Here's how the part is built. I have some questions about the finished solid (model axes, mm). Coordinates: 2 decimals unless noted, no trailing zeros. Order: outer loops, then holes, each group sorted by start corner. A loop starts at its lowest first (then second) coordinate and runs counter-clockwise, first axis right, second up. Notation, with made-up numbers: (24.25, -1) - (83.25, -1) arc R22 ccw to (83.25, 18) - close; hole circle Ø5 at (42, 13.25). An arc over 180 degrees is marked (long way). Answer in a Markdown table with one row per item. Add a question column.
Item 1: I want a section at B-B (y = 1.8). Please give me the cut outline in (x, z) (3 decimals).
Item 2: I want a section at D-D (x = 49). Please give me the cut outline in (y, z) (3 decimals).
Item 3: I want a section at C-C (z = -168). Please give me the cut outline in (x, y) (3 decimals).
Item 4: Will these pins go through, and if not, where does the flat tip stop? pin 1 Ø1 at (y, z) = (1, -153.5) entering from +X; pin 2 Ø1 at (y, z) = (1, -146.5) entering from +X; pin 3 Ø8 at (x, z) = (265.28, -74.56) entering from -Y.
Item 5: I want a section at A-A (x = 224.75). Please give me the cut outline in (y, z) (3 decimals).
Item 6: If I drill on line 1 along Z through (x, y) = (389, 1.45); line 2 along X through (y, z) = (0.75, -97); line 3 along X through (y, z) = (0.65, -95.5), over which ranges is the centre line in solid material (lowest first)? Write a range as from..to.
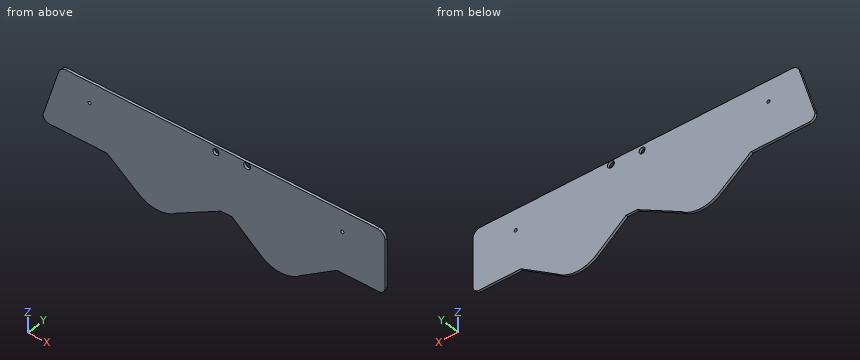
```python
from build123d import *

# Parameters (mm, degrees)
SKETCH1_R           = 3.716178426
SKETCH1_R_2         = 4.313560469
SKETCH1_R_3         = 4.511205791
BOSS_EXTRUDE1_DEPTH = 3.175
SKETCH2_W           = 597.466303312
SKETCH2_H           = 60.972543052
CUT_EXTRUDE1_DEPTH  = 70
FILLET1_R           = 10
FILLET2_R           = 10
SKETCH3_R           = 3.990837639
CUT_EXTRUDE2_DEPTH  = 10
SKETCH4_R           = 2
CUT_EXTRUDE3_DEPTH  = 470.13785887
SKETCH5_R           = 2
CUT_EXTRUDE4_DEPTH  = 10
SKETCH6_R           = 40
BOSS_EXTRUDE2_DEPTH = 3.175
BOSS_EXTRUDE3_DEPTH = 3.175
SKETCH9_R           = 40
BOSS_EXTRUDE4_DEPTH = 3.175
BOSS_EXTRUDE6_DEPTH = 3.175


with BuildPart() as part:
    # Sketch1 → Boss-Extrude1 (new body)
    with BuildSketch(Plane(origin=(0, 0, 0), x_dir=(1, 0, 0), z_dir=(0, 1, 0))):
        with BuildLine():
            ThreePointArc((8, 150), (2.343145751, 147.656854249), (0, 142))
            Line((0, 142), (42, 8))
            ThreePointArc((42, 8), (44.343145751, 2.343145751), (50, 0))
            Line((50, 0), (436.5, 0))
            ThreePointArc((436.5, 0), (442.156854249, 2.343145751), (444.5, 8))
            Line((444.5, 8), (444.5, 142))
            ThreePointArc((444.5, 142), (442.156854249, 147.656854249), (436.5, 150))
            Line((436.5, 150), (8, 150))
        make_face()
        with Locations(Location((146.269370224, 139.84039861, 0), (0, 0, 270))):
            Circle(SKETCH1_R, mode=Mode.SUBTRACT)
        with Locations(Location((307.606475607, 140.710564477, 0), (0, 0, 270))):
            Circle(SKETCH1_R_2, mode=Mode.SUBTRACT)
        with Locations(Location((265.281257274, 74.563866981, 0), (0, 0, 270))):
            Circle(SKETCH1_R_3, mode=Mode.SUBTRACT)
    extrude(amount=BOSS_EXTRUDE1_DEPTH)

    # Sketch2 → Cut-Extrude1 (cut)
    with BuildSketch(Plane.XY):
        with Locations((220.1785332, 7.544358636)):
            Rectangle(SKETCH2_W, SKETCH2_H)
    extrude(amount=-CUT_EXTRUDE1_DEPTH, mode=Mode.SUBTRACT)

    # Fillet1
    fillet1_edges = [part.edges().sort_by_distance(p)[0] for p in [
        (22.567164179, 1.5875, -70),
    ]]
    fillet(fillet1_edges, radius=FILLET1_R)

    # Fillet2
    fillet2_edges = [part.edges().sort_by_distance(p)[0] for p in [
        (444.5, 1.5875, -70),
    ]]
    fillet(fillet2_edges, radius=FILLET2_R)

    # Sketch3 → Cut-Extrude2 (cut)
    with BuildSketch(Plane(origin=(0, 3.175, 0), x_dir=(1, 0, 0), z_dir=(0, 1, 0))):
        with Locations(Location((224.75, 77.255, 0), (0, 0, 270))):
            Circle(SKETCH3_R)
    extrude(amount=-CUT_EXTRUDE2_DEPTH, mode=Mode.SUBTRACT)

    # Sketch4 → Cut-Extrude3 (cut, through all)
    with BuildSketch(Plane(origin=(0, 3.175, 0), x_dir=(1, 0, 0), z_dir=(0, 1, 0))):
        with Locations(Location((60.5, 97, 0), (0, 0, 270))):
            Circle(SKETCH4_R)
    extrude(amount=-CUT_EXTRUDE3_DEPTH, mode=Mode.SUBTRACT)

    # Sketch5 → Cut-Extrude4 (cut)
    with BuildSketch(Plane(origin=(0, 3.175, 0), x_dir=(1, 0, 0), z_dir=(0, 1, 0))):
        with Locations(Location((389, 97, 0), (0, 0, 270))):
            Circle(SKETCH5_R)
    extrude(amount=-CUT_EXTRUDE4_DEPTH, mode=Mode.SUBTRACT)

    # Sketch6 → Boss-Extrude2 (add)
    with BuildSketch(Plane(origin=(0, 0, 0), x_dir=(1, 0, 0), z_dir=(0, 1, 0))):
        with Locations((149, 150.04039861)):
            Circle(SKETCH6_R)
    extrude(amount=BOSS_EXTRUDE2_DEPTH)

    # Sketch7 → Boss-Extrude3 (add)
    with BuildSketch(Plane(origin=(0, 0, 0), x_dir=(1, 0, 0), z_dir=(0, 1, 0))):
        Polygon((124.164543783, 181.396420591), (82.702881078, 149.750534228), (231.468946681, 149.750534228), (173.835456217, 181.396420591), align=None)
    extrude(amount=BOSS_EXTRUDE3_DEPTH)

    # Sketch9 → Boss-Extrude4 (add)
    with BuildSketch(Plane(origin=(0, 0, 0), x_dir=(1, 0, 0), z_dir=(0, 1, 0))):
        with BuildLine():
            ThreePointArc((269, 150), (272.870833001, 167.166341835), (283.734164599, 181.010281545))
            Line((283.734164599, 181.010281545), (245.673378314, 150))
            Line((245.673378314, 150), (269, 150))
        make_face()
        with Locations((309, 150)):
            Circle(SKETCH9_R)
    extrude(amount=BOSS_EXTRUDE4_DEPTH)

    # Sketch12 → Boss-Extrude6 (add)
    with BuildSketch(Plane(origin=(0, 0, 0), x_dir=(1, 0, 0), z_dir=(0, 1, 0))):
        Polygon((326.166341835, 186.129166999), (382.106475607, 150), (340.398839744, 150), align=None)
    extrude(amount=BOSS_EXTRUDE6_DEPTH)


solid = part.part
```
Values follow:
| question | item | result |
|---|---|---|
| 1 | outline | (0, -142) arc R8 ccw to (8, -150) - (83.03, -150) - (124.165, -181.396) arc R40 ccw to (173.835, -181.396) - (231.015, -150) - (245.673, -150) - (283.734, -181.01) arc R40 ccw to (334.871, -180.507) - (382.106, -150) - (436.5, -150) arc R8 ccw to (444.5, -142) - (444.5, -80) arc R10 ccw to (434.5, -70) - (29.913, -70) arc R10 ccw to (20.37, -77.009) - close; hole circle Ø4 at (60.5, -97); hole circle Ø7.982 at (224.75, -77.255); hole circle Ø9.022 at (265.281, -74.564); hole circle Ø4 at (389, -97) |
| 2 | outline | (0, -150) - (3.175, -150) - (3.175, -70) - (0, -70) - close |
| 3 | outline | (106.613, 0) - (198.233, 0) - (198.233, 3.175) - (106.613, 3.175) - close; (267.766, 0) - (354.236, 0) - (354.236, 3.175) - (267.766, 3.175) - close |
| 4 | pin 1 | stops at x = 377.46 |
| 4 | pin 2 | stops at x = 443.43 |
| 4 | pin 3 | passes through |
| 5 | outline | (0, -153.44) - (3.175, -153.44) - (3.175, -81.246) - (0, -81.246) - close; (0, -73.264) - (3.175, -73.264) - (3.175, -70) - (0, -70) - close |
| 6 | line 1 | z = -150..-99, -95..-70 |
| 6 | line 2 | x = 14.1..58.5, 62.5..387, 391..444.5 |
| 6 | line 3 | x = 14.57..59.18, 61.82..387.68, 390.32..444.5 |
